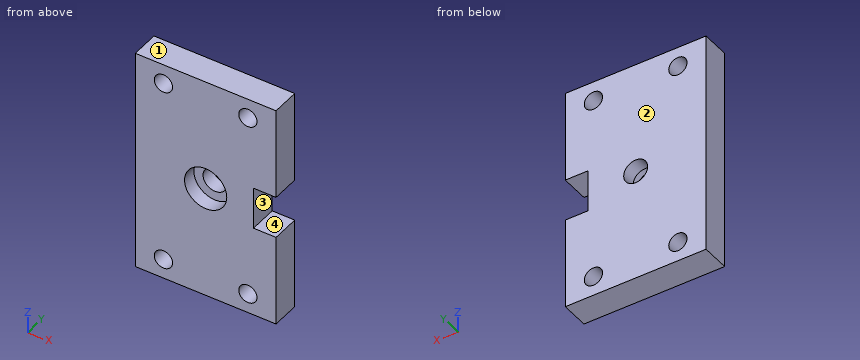
from build123d import *

# Parameters (mm, degrees)
SKETCH1_W           = 50
SKETCH1_H           = 80
BOSS_EXTRUDE1_DEPTH = 10
CUT_EXTRUDE1_REACH  = 12
SKETCH2_R           = 4.25
CUT_EXTRUDE3_REACH  = 12
SKETCH5_R           = 3.25
SKETCH7_R           = 7.5
CUT_EXTRUDE4_DEPTH  = 5
SKETCH10_W          = 8
SKETCH10_H          = 15
CUT_EXTRUDE5_DEPTH  = 11


with BuildPart() as part:
    # Sketch1 → Boss-Extrude1 (new body)
    with BuildSketch(Plane(origin=(0, 0, 0), x_dir=(1, 0, 0), z_dir=(0, 1, 0))):
        with Locations((5.890258642, -6.741379093)):
            Rectangle(SKETCH1_W, SKETCH1_H)
    extrude(amount=BOSS_EXTRUDE1_DEPTH)

    # Sketch2 → Cut-Extrude1 (cut, up to next)
    with BuildSketch(Plane.XZ, mode=Mode.PRIVATE) as cut_extrude1_sk1:
        with Locations((5.890258642, 6.741379093)):
            Circle(SKETCH2_R)
    cut_extrude1_tool1 = extrude(cut_extrude1_sk1.sketch, amount=-CUT_EXTRUDE1_REACH, mode=Mode.PRIVATE) & part.part
    add(cut_extrude1_tool1.solids().sort_by_distance((5.890259, 0, 6.741379))[0], mode=Mode.SUBTRACT)

    # Sketch5 → Cut-Extrude3 (cut, up to next)
    with BuildSketch(Plane(origin=(0, 10, 0), x_dir=(1, 0, 0), z_dir=(0, 1, 0)), mode=Mode.PRIVATE) as cut_extrude3_sk1:
        with Locations((-9.109741358, -39.741379093)):
            Circle(SKETCH5_R)
    cut_extrude3_tool1 = extrude(cut_extrude3_sk1.sketch, amount=-CUT_EXTRUDE3_REACH, mode=Mode.PRIVATE) & part.part
    add(cut_extrude3_tool1.solids().sort_by_distance((-9.109741, 10, 39.741379))[0], mode=Mode.SUBTRACT)
    # Sketch5 → Cut-Extrude3 (cut, up to next)
    with BuildSketch(Plane(origin=(0, 10, 0), x_dir=(1, 0, 0), z_dir=(0, 1, 0)), mode=Mode.PRIVATE) as cut_extrude3_sk2:
        with Locations((20.890258642, -39.741379093)):
            Circle(SKETCH5_R)
    cut_extrude3_tool2 = extrude(cut_extrude3_sk2.sketch, amount=-CUT_EXTRUDE3_REACH, mode=Mode.PRIVATE) & part.part
    add(cut_extrude3_tool2.solids().sort_by_distance((20.890259, 10, 39.741379))[0], mode=Mode.SUBTRACT)
    # Sketch5 → Cut-Extrude3 (cut, up to next)
    with BuildSketch(Plane(origin=(0, 10, 0), x_dir=(1, 0, 0), z_dir=(0, 1, 0)), mode=Mode.PRIVATE) as cut_extrude3_sk3:
        with Locations((-9.109741358, 26.258620907)):
            Circle(SKETCH5_R)
    cut_extrude3_tool3 = extrude(cut_extrude3_sk3.sketch, amount=-CUT_EXTRUDE3_REACH, mode=Mode.PRIVATE) & part.part
    add(cut_extrude3_tool3.solids().sort_by_distance((-9.109741, 10, -26.258621))[0], mode=Mode.SUBTRACT)
    # Sketch5 → Cut-Extrude3 (cut, up to next)
    with BuildSketch(Plane(origin=(0, 10, 0), x_dir=(1, 0, 0), z_dir=(0, 1, 0)), mode=Mode.PRIVATE) as cut_extrude3_sk4:
        with Locations((20.890258642, 26.258620907)):
            Circle(SKETCH5_R)
    cut_extrude3_tool4 = extrude(cut_extrude3_sk4.sketch, amount=-CUT_EXTRUDE3_REACH, mode=Mode.PRIVATE) & part.part
    add(cut_extrude3_tool4.solids().sort_by_distance((20.890259, 10, -26.258621))[0], mode=Mode.SUBTRACT)

    # Sketch7 → Cut-Extrude4 (cut)
    with BuildSketch(Plane.XZ):
        with Locations((5.890258642, 6.741379093)):
            Circle(SKETCH7_R)
    extrude(amount=-CUT_EXTRUDE4_DEPTH, mode=Mode.SUBTRACT)

    # Sketch10 → Cut-Extrude5 (cut, through all)
    with BuildSketch(Plane(origin=(0, 10, 0), x_dir=(1, 0, 0), z_dir=(0, 1, 0))):
        with Locations((26.890258642, -6.741379093)):
            Rectangle(SKETCH10_W, SKETCH10_H)
    extrude(amount=-CUT_EXTRUDE5_DEPTH, mode=Mode.SUBTRACT)


solid = part.part
Design review of the part built by this model. Coordinates are the model's own, in mm. Face numbers are marked on the shaded views. Give positions to 0.01 mm unless a question says otherwise; leave off trailing zeros. Write each loop counter-clockwise with the first axis right and the second up, starting at its lowest first coordinate (ties: lowest second). Pieces come first, ordered by that corner, then holes. Notation, with made-up numbers: M 9.5,63 L 48.5,63 A38 cw 48.5,101 Z; hole C 4,26 d8. An arc over 180 degrees is marked long. Answer as a JSON object with one key per item and string values. Group by question number.
1) We need section D-D (z = 10). Give the boundary of the cut face in (x, y), and give its area (3 significant figures).
2) We need section C-C (x = 22). Give the boundary of the cut face in (y, z), and give its area (3 significant figures).
3) Clearance check with a flat-ended pin moving along its axis: pin 1 Ø3 at (y, z) = (3, 9) entering from +X. State where the tip first meets the part, or that it passes through.
4) We need section B-B (z = 41). Give the boundary of the cut face in (x, y).
5) We need section A-A (x = 27.5). Give the boundary of the cut face in (y, z).
6) For line 1 along Z through (x, y) = (-7.5, 9.75); line 2 along Z through (x, y) = (-9.5, 1.25); line 3 along Z through (x, y) = (28, 9), list the stretches that pass through material, from the lowest coordinate up.
7) Mouldability with a two-part tool opening along Z and no side actions: class the marked faces 1, 2, 3 and 4 as released by +Z, released by -Z, zero draft, split by the parting line, or undercut.
Answer key:
{
 "1": {"outline": "M -19.11,0 L -0.86,0 L -0.86,5 L 3.16,5 L 3.16,10 L -19.11,10 Z; M 8.62,5 L 12.65,5 L 12.65,0 L 22.89,0 L 22.89,10 L 8.62,10 Z", "area": "325 mm²"},
 "2": {"outline": "M 0,-33.26 L 10,-33.26 L 10,-29.31 L 0,-29.31 Z; M 0,-23.2 L 10,-23.2 L 10,36.69 L 0,36.69 Z; M 0,42.8 L 10,42.8 L 10,46.74 L 0,46.74 Z", "area": "678 mm²"},
 "3": {"pin 1": "stops at x = 22.89"},
 "4": {"outline": "M -19.11,0 L -12.11,0 L -12.11,10 L -19.11,10 Z; M -6.11,0 L 17.89,0 L 17.89,10 L -6.11,10 Z; M 23.89,0 L 30.89,0 L 30.89,10 L 23.89,10 Z"},
 "5": {"outline": "M 0,-33.26 L 10,-33.26 L 10,-0.76 L 0,-0.76 Z; M 0,14.24 L 10,14.24 L 10,46.74 L 0,46.74 Z"},
 "6": {"line 1": "z = -33.26 to -29.08, -23.44 to 36.92, 42.56 to 46.74", "line 2": "z = -33.26 to -29.49, -23.03 to 36.51, 42.97 to 46.74", "line 3": "z = -33.26 to -0.76, 14.24 to 46.74"},
 "7": {"face 1": "released by +Z", "face 2": "zero draft", "face 3": "undercut", "face 4": "undercut"}
}
